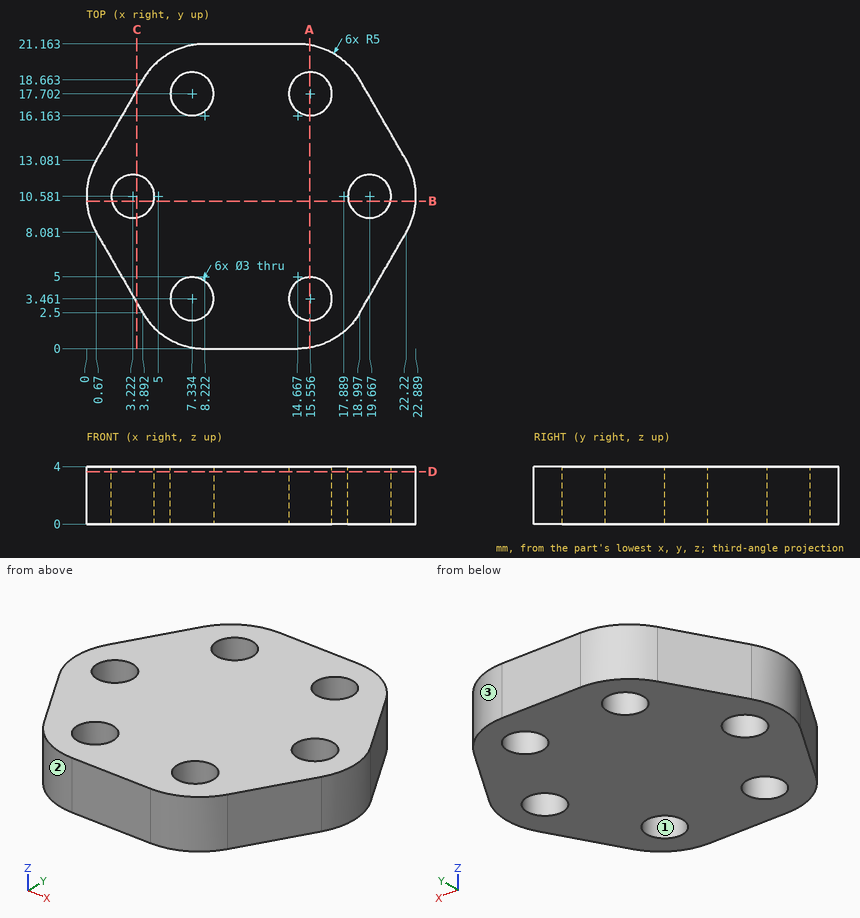
Geometry check sheet. Reference: drawing and pictorial views, mm from the part's lowest x, y, z. Coordinates: 2 decimals unless noted, no trailing zeros. Write each loop counter-clockwise with the first axis right and the second up, starting at its lowest first coordinate (ties: lowest second). Pieces come first, ordered by that corner, then holes. Notation, with made-up numbers: (51, 80) -> (97, 80) arc R28 ccw to (97, 100) -> close; hole circle Ø8 at (78, 68). An arc over 180 degrees is marked (long way). One line per question, with ' | ' between items.
1. Depth check by flat-ended pin: pin 1 Ø1.5 at (y, z) = (15, 2) entering from +X (1 decimal). Enter the tip coordinate at first touch or a pass-through.
Answers:
pin 1: stops at x = 21.5
2. Thickness scan on probe 1 along X at (y, z) = (10.5, 2) (1 decimal); probe 2 along Y at (x, z) = (14.25, 3.4) (1 decimal); probe 3 along X at (y, z) = (11, 3.45). Record the ranges inside material, lowest first. Write a range as from..to.
Answers:
probe 1: x = 0..1.7, 4.7..18.2, 21.2..22.9 | probe 2: y = 0..2.7, 4.2..17, 18.4..21.2 | probe 3: x = 0.02..1.78, 4.66..18.23, 21.11..22.87
3. Cross-section at B-B on y = 10.25. Record the cut outline in (x, z) (1 decimal).
Answers:
outline: (0, 0) -> (1.8, 0) -> (1.8, 4) -> (0, 4) -> close; (4.7, 0) -> (18.2, 0) -> (18.2, 4) -> (4.7, 4) -> close; (21.1, 0) -> (22.9, 0) -> (22.9, 4) -> (21.1, 4) -> close
4. Cross-section at D-D on z = 3.65. Record the cut outline in (x, y) (1 decimal).
Answers:
outline: (0.7, 8.1) -> (3.9, 2.5) arc R5 ccw to (8.2, 0) -> (14.7, 0) arc R5 ccw to (19, 2.5) -> (22.2, 8.1) arc R5 ccw to (22.2, 13.1) -> (19, 18.7) arc R5 ccw to (14.7, 21.2) -> (8.2, 21.2) arc R5 ccw to (3.9, 18.7) -> (0.7, 13.1) arc R5 ccw to start; hole circle Ø3 at (3.2, 10.6); hole circle Ø3 at (7.3, 3.5); hole circle Ø3 at (7.3, 17.7); hole circle Ø3 at (15.6, 3.5); hole circle Ø3 at (15.6, 17.7); hole circle Ø3 at (19.7, 10.6)
5. Cross-section at C-C on x = 3.5. Record the cut outline in (y, z) (1 decimal).
Answers:
outline: (3.2, 0) -> (9.1, 0) -> (9.1, 4) -> (3.2, 4) -> close; (12.1, 0) -> (18, 0) -> (18, 4) -> (12.1, 4) -> close
6. Draft check along X on the marked faces 1, 2 and 3. Enter one of: +X half, -X half, draft (parallel to the pull), parting line (faces both ways), or undercut.
Answers:
face 1: undercut | face 2: -X half | face 3: +X half
7. Cross-section at A-A on x = 15.5. Record the cut outline in (y, z).
Answers:
outline: (0.07, 0) -> (1.96, 0) -> (1.96, 4) -> (0.07, 4) -> close; (4.96, 0) -> (16.2, 0) -> (16.2, 4) -> (4.96, 4) -> close; (19.2, 0) -> (21.09, 0) -> (21.09, 4) -> (19.2, 4) -> close
